```python
from build123d import *

# Parameters (mm, degrees)
F0_R     = 5.08
F1_DEPTH = 50.8
F3_R     = 5.08
F4_DEPTH = 25.0825
F8_W     = 1.2546490179
F8_H     = 6.7444416398
F9_DEPTH = 2.54


with BuildPart() as f1:
    # F0 (on Front) → F1 (new body)
    with BuildSketch(Plane.XZ):
        Circle(F0_R)
    extrude(amount=F1_DEPTH)

    # F3 (on offset) → F4 (join)
    with BuildSketch(Plane.XY.offset(-5.08)):
        with Locations((0, -55.88)):
            Circle(F3_R)
        with Locations((0, 5.08)):
            Circle(F3_R)
    extrude(amount=-F4_DEPTH)

    # F6: sweep along a path in F5
    with BuildLine(Plane.YZ) as f6_path:
        ThreePointArc((5.08, -5.08), (3.5921024484, -1.4878975516), (0, 0))
    # F1_face (on face) → F6 (sweep)
    with BuildSketch(Plane(origin=(0, 0, 0), x_dir=(1, 0, 0), z_dir=(0, 1, 0))):
        with BuildLine():
            ThreePointArc((5.4e-09, 5.08), (-3.5921024504, -3.5921024465), (5.08, 0))
            ThreePointArc((5.08, 0), (3.5921024504, 3.5921024465), (5.4e-09, 5.08))
        make_face()
    sweep(path=f6_path.line)

    # F7: sweep along a path in F5
    with BuildLine(Plane.YZ) as f7_path:
        ThreePointArc((-50.8, 0), (-54.3921024484, -1.4878975516), (-55.88, -5.08))
    # F1_face1 (on face) → F7 (sweep)
    with BuildSketch(Plane.XZ.offset(50.8)):
        with BuildLine():
            ThreePointArc((5.08, 0), (-3.5921024472, 3.5921024497), (-3.5e-09, -5.08))
            ThreePointArc((-3.5e-09, -5.08), (3.5921024472, -3.5921024497), (5.08, 0))
        make_face()
    sweep(path=f7_path.line)

    # F8 (on face) → F9 (cut)
    with BuildSketch(Plane(origin=(0, 0, -30.1625), x_dir=(1, 0, 0), z_dir=(0, 0, -1))):
        with Locations((0, -5.08)):
            Rectangle(F8_W, F8_H)
    extrude(amount=-F9_DEPTH, mode=Mode.SUBTRACT)


solid = f1.part
```
Source: CAD feature listing. Evaluate the final solid. Frame: model axes, mm. A direction names the side the tool comes from. Give positions to 0.01 mm unless a question says otherwise; leave off trailing zeros. Loops run counter-clockwise (first coordinate to the right, second up) from the corner with the lowest first, then second, coordinate; pieces in that order, holes last. Notation, with made-up numbers: M -15.75,11.25 L 11.25,11.25 A16 ccw 11.25,33.25 Z; hole C -30,13.25 d2. An arc over 180 degrees is marked long. Put each result on its own line as item: value.
Q1. Pin query (flat end, axial travel): P1, Ø5, axis at x = -2, y = -20, coming from the -Z side; P2, Ø1.3, axis at y = 4, z = -29.5, coming from the +X side; P3, Ø0.8, axis at y = 4.5, z = -29, coming from the -X side. Return the tip coordinate at first contact, or that it passes through.
Response values:
P1: stops at z = -5.08
P2: stops at x = 5.06
P3: stops at x = -5.08
Q2. Mould query, pull axis X, two halves, no side actions, for faces 4 (the flat face through (0, 1.708, -29)), 5 (the cylindrical face through (-0.661, -50.843, -17.446)), 6 (the flat face through (0, -56, -30.162)). Classes: released by +X, released by -X, zero draft, split by the parting line, or undercut.
Response values:
face 4: undercut
face 5: split by the parting line
face 6: zero draft
Q3. Section A-A (z = -7). Return the cut outline in (x, y).
Response values:
outline: C 0,-55.88 d10.16; C 0,5.08 d10.16
Q4. Section D-D (x = -1.5). Return the cut outline in (y, z).
Response values:
outline: M -60.73,-30.16 L -51.03,-30.16 L -51.03,-5.08 A0.23 cw -50.8,-4.85 L 0,-4.85 A0.23 cw 0.23,-5.08 L 0.23,-30.16 L 9.93,-30.16 L 9.93,-5.08 A9.93 ccw 0,4.85 L -50.8,4.85 A9.93 ccw -60.73,-5.08 Z
Q5. Line query: probe 1 along Y at (x, z) = (4.5, -6.5); probe 2 along Y at (x, z) = (-3.5, -14.5); probe 3 along X at (y, z) = (-23.5, -1). Output: solid intervals per line, ascending. Write a range as [from, to].
Response values:
probe 1: y = [-58.24, -53.52], [2.72, 7.44]
probe 2: y = [-59.56, -52.2], [1.4, 8.76]
probe 3: x = [-4.98, 4.98]
Q6. Section C-C (y = -27.5). Return the cut outline in (x, z).
Response values:
outline: C 0,0 d10.16
Q7. Section B-B (x = 1.75). Return the cut outline in (y, z).
Response values:
outline: M -60.65,-30.16 L -51.11,-30.16 L -51.11,-5.08 A0.31 cw -50.8,-4.77 L 0,-4.77 A0.31 cw 0.31,-5.08 L 0.31,-30.16 L 9.85,-30.16 L 9.85,-5.08 A9.85 ccw 0,4.77 L -50.8,4.77 A9.85 ccw -60.65,-5.08 Z
Q8. Reachability of faces 1 (the flat face through (1, 5, -30.162)), 2 (the cylindrical face through (-0.661, -25.044, 5.037)), 3 (the cylindrical face through (-1.1, 0.12, -17.45)) from +Z, -Z, +X, -X, +Y, -Y: full face, straight path, thin tool, end or side. Return the list, or none.
Response values:
face 1: -Z, +X, -X, +Y, -Y
face 2: none
face 3: -Z
